```python
from build123d import *

# Parameters (mm, degrees)
ESQUISSE1_W             = 140
ESQUISSE1_H             = 30
BOSS_EXTRU_1_DEPTH      = 20
ESQUISSE2_R             = 1
ENL_V_MAT_EXTRU_1_DEPTH = 10
ESQUISSE4_R             = 1
ENL_V_MAT_EXTRU_2_DEPTH = 10
ESQUISSE5_W             = 10
ESQUISSE5_H             = 22
ENL_V_MAT_EXTRU_3_DEPTH = 63
ESQUISSE6_W             = 10
ESQUISSE6_H             = 22
ENL_V_MAT_EXTRU_4_DEPTH = 63
ENL_V_MAT_EXTRU_5_REACH = 83.358
ESQUISSE7_W             = 12
ESQUISSE7_H             = 54.5
ENL_V_MAT_EXTRU_6_REACH = 83.358
ESQUISSE8_W             = 12
ESQUISSE8_H             = 54.5
CONG_1_R                = 2
ESQUISSE9_W             = 54.518801533
ESQUISSE9_H             = 21.792349727
ENL_V_MAT_EXTRU_7_DEPTH = 79.996266608
ESQUISSE11_W            = 54.518801533
ESQUISSE11_H            = 21.792349727
ENL_V_MAT_EXTRU_8_DEPTH = 79.996266608


with BuildPart() as part:
    # Esquisse1 → Boss.-Extru.1 (new body)
    with BuildSketch(Plane(origin=(0, 0, 0), x_dir=(0, 0, -1), z_dir=(1, 0, 0))):
        with Locations((2.932604736, 10.792349727)):
            Rectangle(ESQUISSE1_W, ESQUISSE1_H)
    extrude(amount=BOSS_EXTRU_1_DEPTH)

    # Esquisse2 → Enlèv. mat.-Extru.1 (cut)
    with BuildSketch(Plane(origin=(20, 0, 0), x_dir=(0, 0, -1), z_dir=(1, 0, 0))):
        with Locations((67.832604736, 16.118903051)):
            Circle(ESQUISSE2_R)
        with Locations((17.332604736, 5.818903051)):
            Circle(ESQUISSE2_R)
        Polygon((63.332604736, -0.681096949), (21.332604736, -0.681096949), (21.332604736, 21.318903051), (63.332604736, 21.318903051), (63.332604736, 12.318903051), (63.332604736, 8.068903051), align=None)
    extrude(amount=-ENL_V_MAT_EXTRU_1_DEPTH, mode=Mode.SUBTRACT)

    # Esquisse4 → Enlèv. mat.-Extru.2 (cut)
    with BuildSketch(Plane(origin=(20, 26.612998823, 128.329870586), x_dir=(0, 0, 1), z_dir=(1, 0, 0))):
        with Locations(Location((-117.356713594, 11.320649096, 0), (0, 0, 180))):
            Circle(ESQUISSE4_R)
        with Locations(Location((-66.856713594, 21.620649096, 0), (0, 0, 180))):
            Circle(ESQUISSE4_R)
        Polygon((-113.356713594, 26.820649096), (-113.356713594, 4.820649096), (-71.356713594, 4.820649096), (-71.356713594, 13.570649096), (-71.356713594, 18.070649096), (-71.356713594, 26.820649096), align=None)
    extrude(amount=-ENL_V_MAT_EXTRU_2_DEPTH, mode=Mode.SUBTRACT)

    # Esquisse5 → Enlèv. mat.-Extru.3 (cut)
    with BuildSketch(Plane.XY.offset(67.067395264)):
        with Locations((11, 10.792349727)):
            Rectangle(ESQUISSE5_W, ESQUISSE5_H)
    extrude(amount=-ENL_V_MAT_EXTRU_3_DEPTH, mode=Mode.SUBTRACT)

    # Esquisse6 → Enlèv. mat.-Extru.4 (cut)
    with BuildSketch(Plane(origin=(0, 0, -72.932604736), x_dir=(-1, 0, 0), z_dir=(0, 0, -1))):
        with Locations((-11, 10.792349727)):
            Rectangle(ESQUISSE6_W, ESQUISSE6_H)
    extrude(amount=-ENL_V_MAT_EXTRU_4_DEPTH, mode=Mode.SUBTRACT)

    # Enlèv. mat.-Extru.5: up to this face of the body (flat: up to its plane)
    enl_v_mat_extru_5_end = Plane(part.part.faces().sort_by_distance((11, 21.792349727, -41.432604736))[0])
    # Esquisse7 → Enlèv. mat.-Extru.5 (cut, up to the picked face)
    with BuildSketch(Plane.XZ.offset(4.207650273), mode=Mode.PRIVATE) as enl_v_mat_extru_5_sk1:
        with Locations((10, -37.182604736)):
            Rectangle(ESQUISSE7_W, ESQUISSE7_H)
    enl_v_mat_extru_5_tool1 = split(extrude(enl_v_mat_extru_5_sk1.sketch, amount=-ENL_V_MAT_EXTRU_5_REACH, mode=Mode.PRIVATE), bisect_by=enl_v_mat_extru_5_end, keep=Keep.BOTH, mode=Mode.PRIVATE)
    add(enl_v_mat_extru_5_tool1.solids().sort_by(Axis((10, -4.20765, -37.182605), (0, 1, 0)))[0], mode=Mode.SUBTRACT)

    # Enlèv. mat.-Extru.6: up to this face of the body (flat: up to its plane)
    enl_v_mat_extru_6_end = Plane(part.part.faces().sort_by_distance((12.473684211, 21.792349727, 35.652818786))[0])
    # Esquisse8 → Enlèv. mat.-Extru.6 (cut, up to the picked face)
    with BuildSketch(Plane(origin=(0, -4.207650273, 0), x_dir=(-1, 0, 0), z_dir=(0, -1, 0)), mode=Mode.PRIVATE) as enl_v_mat_extru_6_sk1:
        with Locations((-10, -31.317395264)):
            Rectangle(ESQUISSE8_W, ESQUISSE8_H)
    enl_v_mat_extru_6_tool1 = split(extrude(enl_v_mat_extru_6_sk1.sketch, amount=-ENL_V_MAT_EXTRU_6_REACH, mode=Mode.PRIVATE), bisect_by=enl_v_mat_extru_6_end, keep=Keep.BOTH, mode=Mode.PRIVATE)
    add(enl_v_mat_extru_6_tool1.solids().sort_by(Axis((10, -4.20765, 31.317395), (0, 1, 0)))[0], mode=Mode.SUBTRACT)

    # Congé1
    cong_1_edges = [part.edges().sort_by_distance(p)[0] for p in [
        (4, -4.207650273, -37.182604736),
        (10, -4.207650273, -64.432604736),
        (16, -4.207650273, -37.182604736),
        (10, -4.207650273, -9.932604736),
        (20, 10.792349727, -72.932604736),
        (4, -4.207650273, 31.317395264),
        (10, -4.207650273, 4.067395264),
        (16, -4.207650273, 31.317395264),
        (10, -4.207650273, 58.567395264),
        (20, 25.792349727, -2.932604736),
        (20, 10.792349727, 67.067395264),
        (0, 25.792349727, -2.932604736),
        (0, 10.792349727, -72.932604736),
        (0, -4.207650273, -2.932604736),
        (0, 10.792349727, 67.067395264),
        (11, 21.792349727, 67.067395264),
        (6, 10.792349727, 67.067395264),
        (11, -0.207650273, 67.067395264),
        (16, 10.792349727, 67.067395264),
        (10, 25.792349727, 67.067395264),
        (10, 25.792349727, -72.932604736),
        (10, -4.207650273, -72.932604736),
        (10, -4.207650273, 67.067395264),
        (20, -4.207650273, -2.932604736),
        (11, 21.792349727, -72.932604736),
        (16, 10.792349727, -72.932604736),
        (11, -0.207650273, -72.932604736),
        (6, 10.792349727, -72.932604736),
    ]]
    fillet(cong_1_edges, radius=CONG_1_R - 0.0001)  # a hair under: the kernel refuses the full size

    # Esquisse9 → Enlèv. mat.-Extru.7 (cut, through all)
    with BuildSketch(Plane.ZY.offset(-16)):
        with Locations((31.349786376, 10.896174864)):
            Rectangle(ESQUISSE9_W, ESQUISSE9_H)
    extrude(amount=ENL_V_MAT_EXTRU_7_DEPTH, mode=Mode.SUBTRACT)

    # Esquisse11 → Enlèv. mat.-Extru.8 (cut, through all)
    with BuildSketch(Plane.ZY.offset(-16)):
        with Locations((-37.192905042, 10.412626725)):
            Rectangle(ESQUISSE11_W, ESQUISSE11_H)
    extrude(amount=ENL_V_MAT_EXTRU_8_DEPTH, mode=Mode.SUBTRACT)


solid = part.part
```
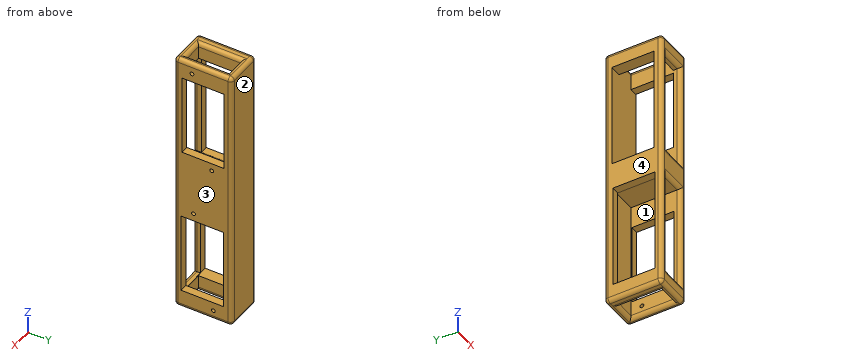
Source: CAD feature listing. Evaluate the final solid. Frame: model axes, mm. Face numbers are marked on the shaded views. Coordinates: 2 decimals unless noted, no trailing zeros. Use a Markdown table: item, result. Add a question column.
Q1. Material intervals for L1, parallel to Z at x = 18.25, y = 11; L2, parallel to Z at x = 2.5, y = 9; L3, parallel to Y at x = 18.25, z = -43.5, sorted ascending.
Q2. Draft query along X for the marked faces 1, 2, 3 and 4. Return one class per face: pulls with the +X half, pulls with the -X half, needs draft (parallel to the pull), parting line crosses it, or undercut.
Q3. First-contact query: pin 1 (7 mm diameter, centred on y = 15, z = 19, fed in from +X); pin 2 (9.5 mm diameter, centred on x = 13, z = -42, fed in from -Y); pin 3 (6 mm diameter, centred on x = 11, z = 43.5, fed in from -Y); pin 4 (0.7 mm diameter, centred on x = 10, y = -1.5, fed in from -Z). Flat tips, straight axial feed; report the tip coordinate or a pass-through.
Q4. Section query A-A, the plane z = -27.5. State how many separate pieces and enclosed holes the cut face has, and give its area (3 significant figures).
Result:
| question | item | result |
|---|---|---|
| 1 | L1 | z = -72.92 to -63.33, -21.33 to 14.97, 56.97 to 67.05 |
| 1 | L2 | z = -72.93 to -64.45, -9.93 to 4.09, 58.61 to 67.07 |
| 1 | L3 | y = -4.19 to -0.68, 21.32 to 25.78 |
| 2 | face 1 | undercut |
| 2 | face 2 | needs draft |
| 2 | face 3 | pulls with the +X half |
| 2 | face 4 | pulls with the -X half |
| 3 | pin 1 | passes through |
| 3 | pin 2 | stops at y = -4.19 |
| 3 | pin 3 | stops at y = 21.79 |
| 3 | pin 4 | stops at z = -72.9 |
| 4 | separate pieces | 3 |
| 4 | enclosed holes | 0 |
| 4 | area | 108 mm2 |
